from build123d import *

# Parameters (mm, degrees)
BASE_FLANGE1_DEPTH            = 1
EDGE_FLANGE1_STRIP_W          = 6
EDGE_FLANGE1_STRIP_H          = 1
EDGE_FLANGE1_STRIP_CUT_DEPTH  = 1158
EDGE_FLANGE1_RELIEF_W         = 6.5
EDGE_FLANGE1_RELIEF_H         = 0.5
EDGE_FLANGE1_RELIEF_CUT_DEPTH = 1
EDGE_FLANGE1_DEPTH            = 1158
EDGE_FLANGE1_PROFILE_W        = 1158
EDGE_FLANGE1_PROFILE_H        = 17
EDGE_FLANGE1_PROFILE_R        = 2.75
EDGE_FLANGE1_FLAT_DEPTH       = 1
CUT_EXTRUDE1_DEPTH            = 10
CUT_EXTRUDE2_DEPTH            = 10


# Sheet-metal steps are written as plain solids
with BuildPart() as part:
    # Sketch1 → Base-Flange1 (new body)
    with BuildSketch(Plane.XY):
        with BuildLine():
            Line((0, 0), (1244, 0))
            Line((1244, 0), (1244, 844))
            ThreePointArc((1244, 844), (1239.313708499, 855.313708499), (1228, 860))
            Line((1228, 860), (16, 860))
            ThreePointArc((16, 860), (4.686291501, 855.313708499), (0, 844))
            Line((0, 844), (0, 0))
        make_face()
    extrude(amount=-BASE_FLANGE1_DEPTH)

    # Edge-Flange1 strip (across the edge) → Edge-Flange1 strip cut (cut)
    with BuildSketch(Plane(origin=(1201, 0, -1), x_dir=(0, 1, 0), z_dir=(-1, 0, 0))):
        with Locations((-1, -0.5)):
            Rectangle(EDGE_FLANGE1_STRIP_W, EDGE_FLANGE1_STRIP_H)
    extrude(amount=EDGE_FLANGE1_STRIP_CUT_DEPTH, mode=Mode.SUBTRACT)

    # Edge-Flange1 relief (on the sheet) → Edge-Flange1 relief cut (cut)
    with BuildSketch(Plane(origin=(1201, 2, -1), x_dir=(0, 1, 0), z_dir=(0, 0, -1))):
        with Locations((-2.75, 0.25)):
            Rectangle(EDGE_FLANGE1_RELIEF_W, EDGE_FLANGE1_RELIEF_H)
        with Locations((-2.75, -1158.25)):
            Rectangle(EDGE_FLANGE1_RELIEF_W, EDGE_FLANGE1_RELIEF_H)
    extrude(amount=-EDGE_FLANGE1_RELIEF_CUT_DEPTH, mode=Mode.SUBTRACT)

    # Edge-Flange1 bend section (across the edge) → Edge-Flange1 (add)
    with BuildSketch(Plane(origin=(1201, 0, -1), x_dir=(0, 1, 0), z_dir=(-1, 0, 0))):
        with BuildLine():
            Line((0, 1), (1, 1))
            ThreePointArc((1, 1), (1.292893219, 0.292893219), (2, 0))
            Line((2, 0), (2, -1))
            ThreePointArc((2, -1), (0.585786438, -0.414213562), (0, 1))
        make_face()
    extrude(amount=EDGE_FLANGE1_DEPTH)

    # Edge-Flange1 profile (on flange) → Edge-Flange1 flat (add)
    with BuildSketch(Plane(origin=(0, 0, -1), x_dir=(-1, 0, 0), z_dir=(0, -1, 0))):
        with Locations((-622, 9.5)):
            Rectangle(EDGE_FLANGE1_PROFILE_W, EDGE_FLANGE1_PROFILE_H)
        with Locations((-802, 9)):
            Circle(EDGE_FLANGE1_PROFILE_R, mode=Mode.SUBTRACT)
        with Locations((-982, 9)):
            Circle(EDGE_FLANGE1_PROFILE_R, mode=Mode.SUBTRACT)
        with Locations((-1162, 9)):
            Circle(EDGE_FLANGE1_PROFILE_R, mode=Mode.SUBTRACT)
        with Locations((-82, 9)):
            Circle(EDGE_FLANGE1_PROFILE_R, mode=Mode.SUBTRACT)
        with Locations((-262, 9)):
            Circle(EDGE_FLANGE1_PROFILE_R, mode=Mode.SUBTRACT)
        with Locations((-442, 9)):
            Circle(EDGE_FLANGE1_PROFILE_R, mode=Mode.SUBTRACT)
        with Locations((-622, 9)):
            Circle(EDGE_FLANGE1_PROFILE_R, mode=Mode.SUBTRACT)
    extrude(amount=-EDGE_FLANGE1_FLAT_DEPTH)

    # Sketch9 → Cut-Extrude1 (cut)
    with BuildSketch(Plane.XY):
        with BuildLine():
            Line((1142.5, 751), (881.5, 751))
            ThreePointArc((881.5, 751), (880.085786438, 750.414213562), (879.5, 749))
            Line((879.5, 749), (879.5, 667))
            ThreePointArc((879.5, 667), (880.085786438, 665.585786438), (881.5, 665))
            Line((881.5, 665), (1142.5, 665))
            ThreePointArc((1142.5, 665), (1143.914213562, 665.585786438), (1144.5, 667))
            Line((1144.5, 667), (1144.5, 749))
            ThreePointArc((1144.5, 749), (1143.914213562, 750.414213562), (1142.5, 751))
        make_face()
        with BuildLine():
            Line((754.5, 749), (754.5, 667))
            ThreePointArc((754.5, 667), (753.914213562, 665.585786438), (752.5, 665))
            Line((752.5, 665), (491.5, 665))
            ThreePointArc((491.5, 665), (490.085786438, 665.585786438), (489.5, 667))
            Line((489.5, 667), (489.5, 749))
            ThreePointArc((489.5, 749), (490.085786438, 750.414213562), (491.5, 751))
            Line((491.5, 751), (752.5, 751))
            ThreePointArc((752.5, 751), (753.914213562, 750.414213562), (754.5, 749))
        make_face()
        with BuildLine():
            Line((364.5, 749), (364.5, 667))
            ThreePointArc((364.5, 667), (363.914213562, 665.585786438), (362.5, 665))
            Line((362.5, 665), (101.5, 665))
            ThreePointArc((101.5, 665), (100.085786438, 665.585786438), (99.5, 667))
            Line((99.5, 667), (99.5, 749))
            ThreePointArc((99.5, 749), (100.085786438, 750.414213562), (101.5, 751))
            Line((101.5, 751), (362.5, 751))
            ThreePointArc((362.5, 751), (363.914213562, 750.414213562), (364.5, 749))
        make_face()
        with BuildLine():
            Line((364.5, 569), (364.5, 487))
            ThreePointArc((364.5, 487), (363.914213562, 485.585786438), (362.5, 485))
            Line((362.5, 485), (101.5, 485))
            ThreePointArc((101.5, 485), (100.085786438, 485.585786438), (99.5, 487))
            Line((99.5, 487), (99.5, 569))
            ThreePointArc((99.5, 569), (100.085786438, 570.414213562), (101.5, 571))
            Line((101.5, 571), (362.5, 571))
            ThreePointArc((362.5, 571), (363.914213562, 570.414213562), (364.5, 569))
        make_face()
        with BuildLine():
            Line((364.5, 389), (364.5, 307))
            ThreePointArc((364.5, 307), (363.914213562, 305.585786438), (362.5, 305))
            Line((362.5, 305), (101.5, 305))
            ThreePointArc((101.5, 305), (100.085786438, 305.585786438), (99.5, 307))
            Line((99.5, 307), (99.5, 389))
            ThreePointArc((99.5, 389), (100.085786438, 390.414213562), (101.5, 391))
            Line((101.5, 391), (362.5, 391))
            ThreePointArc((362.5, 391), (363.914213562, 390.414213562), (364.5, 389))
        make_face()
        with BuildLine():
            Line((754.5, 209), (754.5, 127))
            ThreePointArc((754.5, 127), (753.914213562, 125.585786438), (752.5, 125))
            Line((752.5, 125), (491.5, 125))
            ThreePointArc((491.5, 125), (490.085786438, 125.585786438), (489.5, 127))
            Line((489.5, 127), (489.5, 209))
            ThreePointArc((489.5, 209), (490.085786438, 210.414213562), (491.5, 211))
            Line((491.5, 211), (752.5, 211))
            ThreePointArc((752.5, 211), (753.914213562, 210.414213562), (754.5, 209))
        make_face()
        with BuildLine():
            Line((364.5, 209), (364.5, 127))
            ThreePointArc((364.5, 127), (363.914213562, 125.585786438), (362.5, 125))
            Line((362.5, 125), (101.5, 125))
            ThreePointArc((101.5, 125), (100.085786438, 125.585786438), (99.5, 127))
            Line((99.5, 127), (99.5, 209))
            ThreePointArc((99.5, 209), (100.085786438, 210.414213562), (101.5, 211))
            Line((101.5, 211), (362.5, 211))
            ThreePointArc((362.5, 211), (363.914213562, 210.414213562), (364.5, 209))
        make_face()
        with BuildLine():
            Line((1144.5, 569), (1144.5, 487))
            ThreePointArc((1144.5, 487), (1143.914213562, 485.585786438), (1142.5, 485))
            Line((1142.5, 485), (881.5, 485))
            ThreePointArc((881.5, 485), (880.085786438, 485.585786438), (879.5, 487))
            Line((879.5, 487), (879.5, 569))
            ThreePointArc((879.5, 569), (880.085786438, 570.414213562), (881.5, 571))
            Line((881.5, 571), (1142.5, 571))
            ThreePointArc((1142.5, 571), (1143.914213562, 570.414213562), (1144.5, 569))
        make_face()
        with BuildLine():
            Line((1144.5, 389), (1144.5, 307))
            ThreePointArc((1144.5, 307), (1143.914213562, 305.585786438), (1142.5, 305))
            Line((1142.5, 305), (881.5, 305))
            ThreePointArc((881.5, 305), (880.085786438, 305.585786438), (879.5, 307))
            Line((879.5, 307), (879.5, 389))
            ThreePointArc((879.5, 389), (880.085786438, 390.414213562), (881.5, 391))
            Line((881.5, 391), (1142.5, 391))
            ThreePointArc((1142.5, 391), (1143.914213562, 390.414213562), (1144.5, 389))
        make_face()
        with BuildLine():
            Line((1144.5, 209), (1144.5, 127))
            ThreePointArc((1144.5, 127), (1143.914213562, 125.585786438), (1142.5, 125))
            Line((1142.5, 125), (881.5, 125))
            ThreePointArc((881.5, 125), (880.085786438, 125.585786438), (879.5, 127))
            Line((879.5, 127), (879.5, 209))
            ThreePointArc((879.5, 209), (880.085786438, 210.414213562), (881.5, 211))
            Line((881.5, 211), (1142.5, 211))
            ThreePointArc((1142.5, 211), (1143.914213562, 210.414213562), (1144.5, 209))
        make_face()
    extrude(amount=-CUT_EXTRUDE1_DEPTH, mode=Mode.SUBTRACT)

    # Sketch10 → Cut-Extrude2 (cut)
    with BuildSketch(Plane.XY):
        with BuildLine():
            Line((482, 306.5), (762, 306.5))
            ThreePointArc((762, 306.5), (769.071067812, 309.428932188), (772, 316.5))
            Line((772, 316.5), (772, 561.5))
            ThreePointArc((772, 561.5), (769.071067812, 568.571067812), (762, 571.5))
            Line((762, 571.5), (482, 571.5))
            ThreePointArc((482, 571.5), (474.928932188, 568.571067812), (472, 561.5))
            Line((472, 561.5), (472, 316.5))
            ThreePointArc((472, 316.5), (474.928932188, 309.428932188), (482, 306.5))
        make_face()
    extrude(amount=-CUT_EXTRUDE2_DEPTH, mode=Mode.SUBTRACT)


solid = part.part
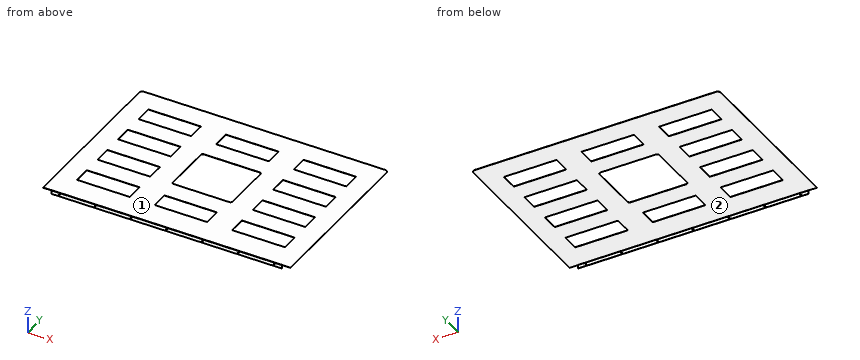
Design review of the part built by this model. Coordinates are the model's own, in mm. Face numbers are marked on the shaded views. Give positions to 0.01 mm unless a question says otherwise; leave off trailing zeros. Loops run counter-clockwise (first coordinate to the right, second up) from the corner with the lowest first, then second, coordinate; pieces in that order, holes last. Notation, with made-up numbers: M 36.5,87 L 64.5,87 A28 cw 64.5,123 Z; hole C 63,2 d6. An arc over 180 degrees is marked long. One line per question, with ' | ' between items. Start each with the question number.
1. The part is to be moulded in two halves that separate along Z. For the marked faces 1 and 2, say which applies: released by +Z, released by -Z, zero draft, split by the parting line, or undercut.
2. Add section C-C (y = 531). Write out the cut boundary in (x, z).
3. To check wall thickness, follow L1, parallel to Z at x = 802, y = 0.45; L2, parallel to Y at x = 774.5, z = -13; L3, parallel to Z at x = 103, y = 759. State the ranges of each line that lie inside material, in increasing order.
4. Insertion check: P1, Ø1.1, axis at x = 588.5, z = -0.5, coming from the -Y side; P2, Ø9, axis at x = 982, z = -10, coming from the -Y side; P3, Ø6, axis at x = 867.5, y = 249.5, coming from the -Z side; P4, Ø0.5, axis at x = 975.5, z = -0.5, coming from the -Y side. Each pin has a flat end and moves straight along its axis. Give the tip position at first contact, or say it passes through.
5. Add section D-D (y = 53). Write out the cut boundary in (x, z), plus the area to 3 significant figures.
6. Add section A-A (y = 188). Write out the cut boundary in (x, z).
7. Add section B-B (x = 967). Write out the cut boundary in (y, z).
Worked out:
1) face 1: released by +Z | face 2: released by -Z
2) outline: M 0,-1 L 99.5,-1 L 99.5,0 L 0,0 Z; M 364.5,-1 L 472,-1 L 472,0 L 364.5,0 Z; M 772,-1 L 879.5,-1 L 879.5,0 L 772,0 Z; M 1144.5,-1 L 1244,-1 L 1244,0 L 1144.5,0 Z
3) L1: z = -19 to -12.75, -7.25 to -0.74 | L2: y = 0 to 1 | L3: z = -1 to 0
4) P1: stops at y = 0.24 | P2: stops at y = 0 | P3: stops at z = -1 | P4: stops at y = 0.44
5) outline: M 0,-1 L 1244,-1 L 1244,0 L 0,0 Z | area: 1,240 mm²
6) outline: M 0,-1 L 99.5,-1 L 99.5,0 L 0,0 Z; M 364.5,-1 L 489.5,-1 L 489.5,0 L 364.5,0 Z; M 754.5,-1 L 879.5,-1 L 879.5,0 L 754.5,0 Z; M 1144.5,-1 L 1244,-1 L 1244,0 L 1144.5,0 Z
7) outline: M 0,-19 L 1,-19 L 1,-2 A1 cw 2,-1 L 125,-1 L 125,0 L 2,0 A2 ccw 0,-2 Z; M 211,-1 L 305,-1 L 305,0 L 211,0 Z; M 391,-1 L 485,-1 L 485,0 L 391,0 Z; M 571,-1 L 665,-1 L 665,0 L 571,0 Z; M 751,-1 L 860,-1 L 860,0 L 751,0 Z
